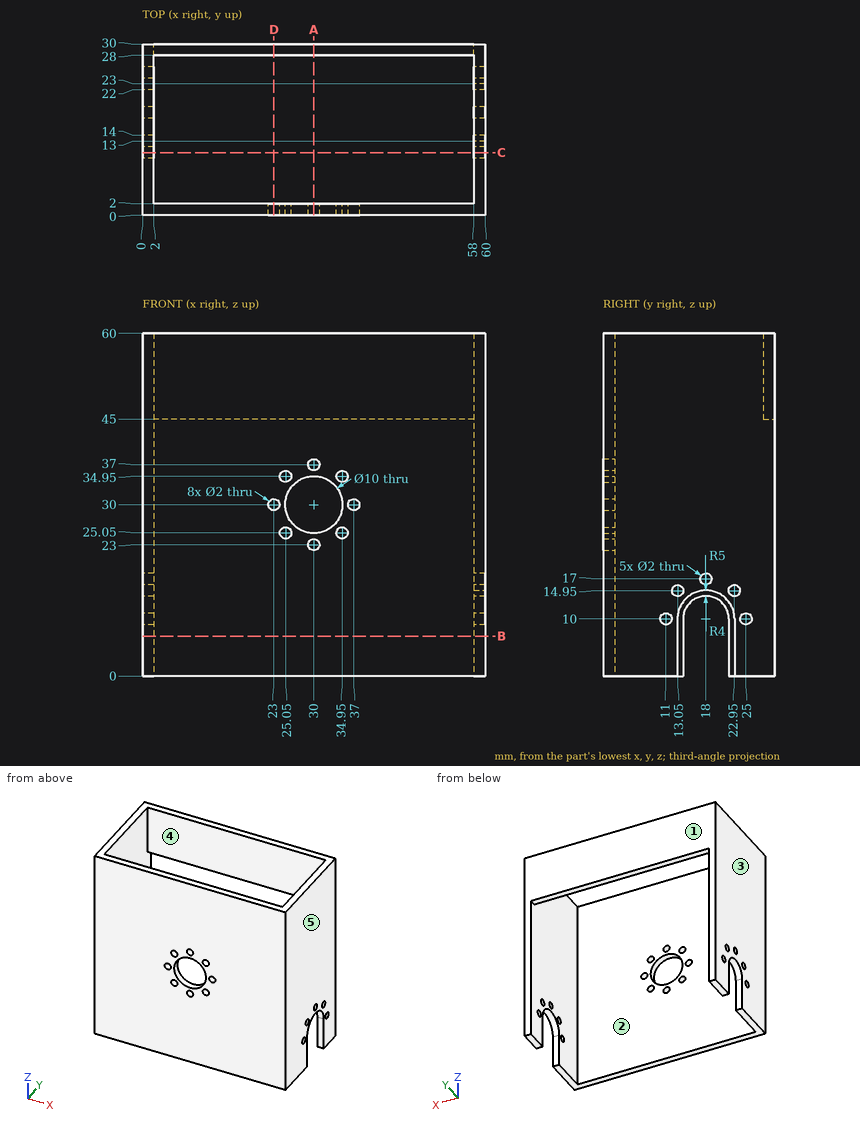
Geometry check sheet. Reference: drawing and pictorial views, mm from the part's lowest x, y, z. A direction names the side the tool comes from. Give positions to 0.01 mm unless a question says otherwise; leave off trailing zeros. Order: outer loops, then holes, each group sorted by start corner. A loop starts at its lowest first (then second) coordinate and runs counter-clockwise, first axis right, second up. Notation, with made-up numbers: (21, 30.5) - (30, 30.5) arc R9 ccw to (30, 37.5) - close; hole circle Ø3 at (11.5, 33). An arc over 180 degrees is marked (long way). Answer as CSV lines item,"result".
1. Go/stop test with flat-tipped pins: P1, Ø2.5, axis at x = 37, z = 30, coming from the +Y side; P2, Ø10, axis at y = 16, z = 52, coming from the -X side; P3, Ø2, axis at x = 33.5, y = 29, coming from the -Z side. Record where each tip stops, or that it passes through.
Result sheet:
P1,"y = 2"
P2,"x = 0"
P3,"z = 45"
2. Scan lines: probe 1 along Y at (x, z) = (11.5, 46.5); probe 2 along X at (y, z) = (11.75, 56.5); probe 3 along Y at (x, z) = (59.25, 10). Record each from-to range of solid material in increasing order. Write a range as from..to.
Result sheet:
probe 1,"0..2, 28..30"
probe 2,"0..2, 58..60"
probe 3,"0..10, 12..13, 23..24, 26..30"
3. Section check A-A (x = 30). Record the boundary of the cut face in (y, z).
Result sheet:
outline,"(0, 0) - (2, 0) - (2, 22) - (0, 22) - close; (0, 24) - (2, 24) - (2, 25) - (0, 25) - close; (0, 35) - (2, 35) - (2, 36) - (0, 36) - close; (0, 38) - (2, 38) - (2, 60) - (0, 60) - close; (28, 45) - (30, 45) - (30, 60) - (28, 60) - close"
4. Tool access check on the marked faces 4 and 5. Record the directions out of +Z, -Z, +X, -X, +Y, -Y that give a thin tool (end or side, any length) a straight path to the whole face; none if there is none.
Result sheet:
face 4,"+Z, -Z"
face 5,"+Z, -Z, +X, +Y, -Y"
5. Section check D-D (x = 23). Record the boundary of the cut face in (y, z).
Result sheet:
outline,"(0, 0) - (2, 0) - (2, 29) - (0, 29) - close; (0, 31) - (2, 31) - (2, 60) - (0, 60) - close; (28, 45) - (30, 45) - (30, 60) - (28, 60) - close"
6. Mould release check, pull along X, two halves, no side actions. Record for the marked faces 1, 2 and 3: released by +X, released by -X, zero draft, split by the parting line, or undercut.
Result sheet:
face 1,"zero draft"
face 2,"undercut"
face 3,"released by -X"
7. Section check B-B (z = 7). Record the boundary of the cut face in (x, y), then the cut area to 3 significant figures.
Result sheet:
outline,"(0, 0) - (60, 0) - (60, 13) - (58, 13) - (58, 2) - (2, 2) - (2, 14) - (0, 14) - close; (0, 22) - (2, 22) - (2, 30) - (0, 30) - close; (58, 23) - (60, 23) - (60, 30) - (58, 30) - close"
area,"196 mm²"
8. Section check C-C (y = 11). Record the boundary of the cut face in (x, z).
Result sheet:
outline,"(0, 0) - (2, 0) - (2, 9) - (0, 9) - close; (0, 11) - (2, 11) - (2, 60) - (0, 60) - close; (58, 0) - (60, 0) - (60, 9) - (58, 9) - close; (58, 11) - (60, 11) - (60, 60) - (58, 60) - close"
